from build123d import *

# Parameters (mm, degrees)
F0_W     = 76.2
F0_H     = 76.2
F1_DEPTH = 19.05
F4_D     = 12.7
F4_DEPTH = 609.6


with BuildPart() as f1:
    # F0 (on Front) → F1 (new body, symmetric)
    with BuildSketch(Plane.XZ):
        Rectangle(F0_W, F0_H)
    extrude(amount=F1_DEPTH, both=True)

    # F4
    with Locations(Plane.XZ.offset(25.38984)):
        with Locations((0, 0)):
            Hole(F4_D / 2, depth=F4_DEPTH)


solid = f1.part
The listing builds one solid part. Answer for the finished solid, in the listing's coordinates (mm). Give positions to 0.01 mm unless a question says otherwise; leave off trailing zeros. Write each loop counter-clockwise with the first axis right and the second up, starting at its lowest first coordinate (ties: lowest second). Pieces come first, ordered by that corner, then holes. Notation, with made-up numbers: (-12, 82) - (34, 82) arc R15 cw to (34, 86) - close; hole circle Ø7 at (26.5, -14.75). An arc over 180 degrees is marked (long way). Use a Markdown table: item, result.
1. Section A-A on z = 0 is taken. Write down the section's boundary in (x, y).
Values follow:
| item | result |
|---|---|
| outline | (-38.1, -19.05) - (-6.35, -19.05) - (-6.35, 19.05) - (-38.1, 19.05) - close; (6.35, -19.05) - (38.1, -19.05) - (38.1, 19.05) - (6.35, 19.05) - close |
2. Section C-C on y = 17 is taken. Write down the section's boundary in (x, z).
Values follow:
| item | result |
|---|---|
| outline | (-38.1, -38.1) - (38.1, -38.1) - (38.1, 38.1) - (-38.1, 38.1) - close; hole circle Ø12.7 at (0, 0) |
3. For a pull along Z with two mould halves and no side action, classify faces 1 (the flat face through (-1, 0, 38.1)), 2 (the flat face through (-1, 0, -38.1)), 3 (the cylindrical face through (1.38, 0.27, -6.2)) as released by +Z, released by -Z, zero draft, split by the parting line, or undercut.
Values follow:
| item | result |
|---|---|
| face 1 | released by +Z |
| face 2 | released by -Z |
| face 3 | undercut |
4. Section B-B on x = 0 is taken. Write down the section's boundary in (y, z).
Values follow:
| item | result |
|---|---|
| outline | (-19.05, -38.1) - (19.05, -38.1) - (19.05, -6.35) - (-19.05, -6.35) - close; (-19.05, 6.35) - (19.05, 6.35) - (19.05, 38.1) - (-19.05, 38.1) - close |
5. This flat-tipped pin is pushed along its axis until it touches: P1, Ø10, axis at x = 0, z = 0, coming from the +Y side. Where does it stop, or does it pass through?
Values follow:
| item | result |
|---|---|
| P1 | passes through |
6. Find the intervals of material crossed by probe 1 along Z at (x, y) = (0, -2); probe 2 along X at (y, z) = (-1.5, -5); probe 3 along Z at (x, y) = (-3.5, -16), in increasing order. Write a range as from..to.
Values follow:
| item | result |
|---|---|
| probe 1 | z = -38.1..-6.35, 6.35..38.1 |
| probe 2 | x = -38.1..-3.91, 3.91..38.1 |
| probe 3 | z = -38.1..-5.3, 5.3..38.1 |
